The drawing under review shows one solid part. Ordinate dimensions are in mm from its lowest x, y, z. Coordinates: 2 decimals unless noted, no trailing zeros. Loops run counter-clockwise (first coordinate to the right, second up) from the corner with the lowest first, then second, coordinate; pieces in that order, holes last. Notation, with made-up numbers: (-35, 13.5) -> (-10, 13.5) arc R31 cw to (-10, 41.5) -> close; hole circle Ø8 at (-10.5, -2). An arc over 180 degrees is marked (long way). Use a Markdown table: item, result.
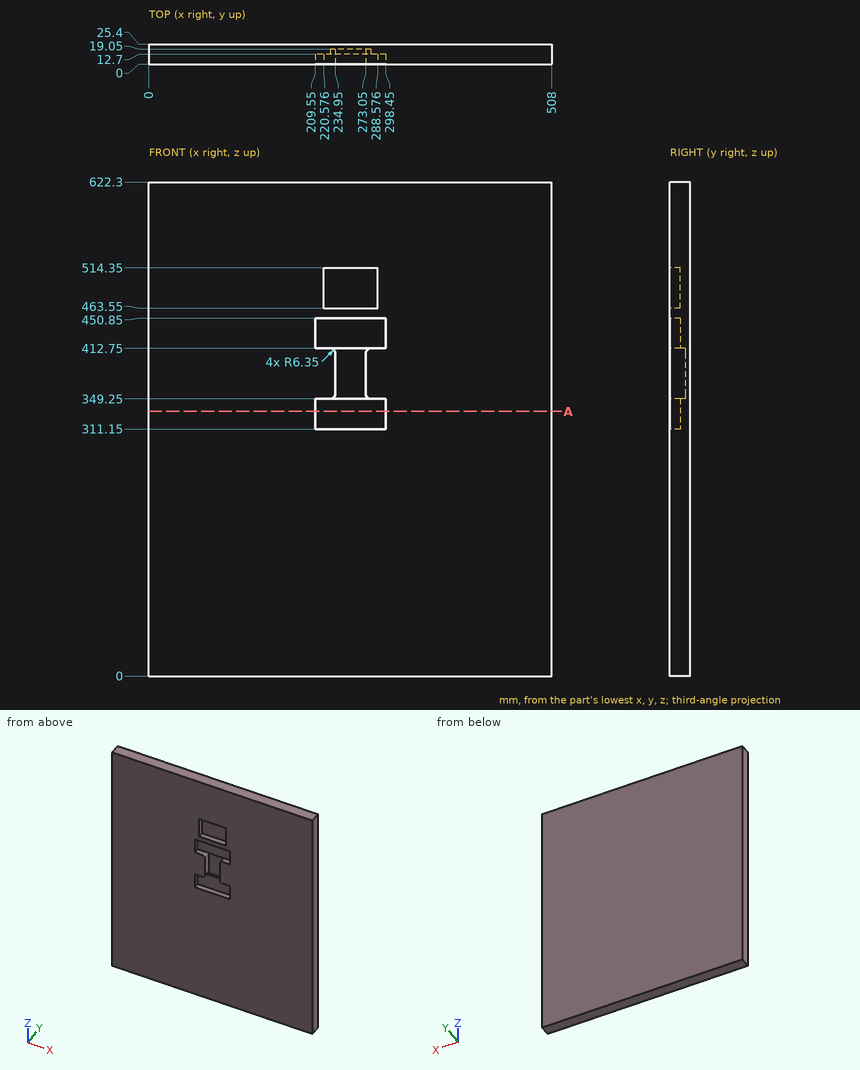
(1) For pin 1 Ø11.5 at (x, z) = (245, 321.5) entering from -Y, flat-tipped, find the tip position at first contact; note if it passes through.
Found:
| item | result |
|---|---|
| pin 1 | stops at y = 12.7 |
(2) Take a section at A-A on z = 333.5. Write out the cut boundary in (x, y), plus the area to 3 significant figures.
Found:
| item | result |
|---|---|
| outline | (0, 0) -> (209.55, 0) -> (209.55, 12.7) -> (298.45, 12.7) -> (298.45, 0) -> (508, 0) -> (508, 25.4) -> (0, 25.4) -> close |
| area | 11,800 mm^2 |
(3) For line 1 along X through (y, z) = (12, 412); line 2 along Y through (x, z) = (253, 450), list the stretches that pass through material, from the lowest coordinate up.
Found:
| item | result |
|---|---|
| line 1 | x = 0 to 231.59, 276.41 to 508 |
| line 2 | y = 12.7 to 25.4 |
